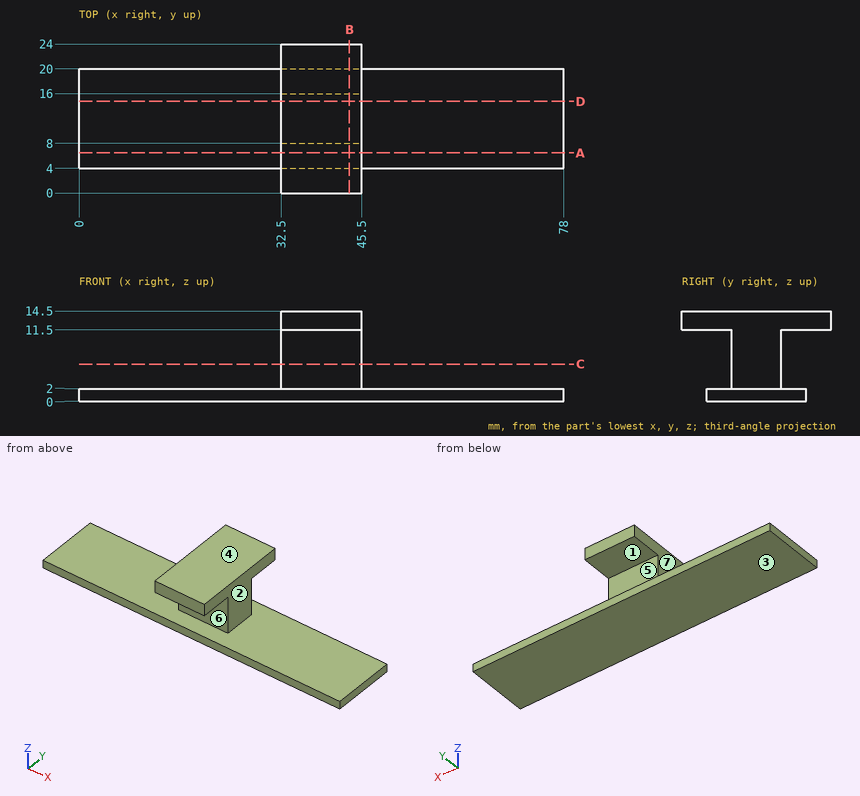
Could you check a few things on this drawing? It's one solid part, dimensions in mm from its lowest x, y, z. A direction names the side the tool comes from. Round coordinates to 2 decimals unless told otherwise and drop trailing zeros. Order: outer loops, then holes, each group sorted by start corner. A loop starts at its lowest first (then second) coordinate and runs counter-clockwise, first axis right, second up. Notation, with made-up numbers: M 38,36.25 L 60,36.25 A19 cw 60,73.25 Z; hole C -14,81 d2. An arc over 180 degrees is marked long. One line per question, with ' | ' between items. Start each with the question number.
(1) Suppose I cut it at B-B on x = 43.5. List the corners of the cut face in (y, z) for me, then the cut area to 3 significant figures.
(2) Suppose I cut it at C-C on z = 6. List the corners of the cut face in (x, y) for me.
(3) Suppose I cut it at A-A on y = 6.5. List the corners of the cut face in (x, z) for me.
(4) For the marked faces 1, 2 and 3, which set-ups out of +Z, -Z, +X, -X, +Y, -Y let a thin tool reach every point of the face, with its end or its side?
(5) Thinking about a two-plate mould opening in Z: for the marked faces 4, 5, 6 and 7, which applies, +Z half, -Z half, draft (parallel to the pull), parting line (faces both ways), or undercut?
(6) For P1, Ø4, axis at y = 15, z = 6, coming from the -X side; P2, Ø4, axis at x = 26.5, z = 3, coming from the -Y side; P3, Ø3, axis at y = 14.5, z = 6, coming from the +X side, each with a flat end and sliding along its axis, tell me the tip position at first contact or that it passes through.
(7) Suppose I cut it at D-D on y = 14.75. List the corners of the cut face in (x, z) for me, then the cut area to 4 significant figures.
(8) Please list where these lines run through material, in increasing order: line 1 along Z through (x, y) = (35.5, 17.25); line 2 along X through (y, z) = (15, 8); line 3 along Z through (x, y) = (49.5, 8.75).
Geometry results:
1) outline: M 0,11.5 L 8,11.5 L 8,2 L 4,2 L 4,0 L 20,0 L 20,2 L 16,2 L 16,11.5 L 24,11.5 L 24,14.5 L 0,14.5 Z | area: 180 mm²
2) outline: M 32.5,8 L 45.5,8 L 45.5,16 L 32.5,16 Z
3) outline: M 0,0 L 78,0 L 78,2 L 0,2 Z; M 32.5,11.5 L 45.5,11.5 L 45.5,14.5 L 32.5,14.5 Z
4) face 1: +X, -X, +Y | face 2: +Z, +X, +Y, -Y | face 3: -Z, +X, -X, +Y, -Y
5) face 4: +Z half | face 5: undercut | face 6: undercut | face 7: draft
6) P1: x = 32.5 | P2: y = 4 | P3: x = 45.5
7) outline: M 0,0 L 78,0 L 78,2 L 45.5,2 L 45.5,14.5 L 32.5,14.5 L 32.5,2 L 0,2 Z | area: 318.5 mm²
8) line 1: 0 to 2, 11.5 to 14.5 | line 2: 32.5 to 45.5 | line 3: 0 to 2
